Here's how the part is built. I have some questions about the finished solid (model axes, mm). Face numbers are marked on the shaded views. Coordinates: 2 decimals unless noted, no trailing zeros. Write each loop counter-clockwise with the first axis right and the second up, starting at its lowest first coordinate (ties: lowest second). Pieces come first, ordered by that corner, then holes. Notation, with made-up numbers: (73, 74) -> (80, 74) arc R20 cw to (80, 83) -> close; hole circle Ø6 at (23, 59). An arc over 180 degrees is marked (long way). Put each result on its own line as item: value. Start each with the question number.
Item 1: For pin 1 (3.5 mm diameter, centred on x = 9, z = -5.5, fed in from -Y), with a flat end and sliding along its axis, tell me the tip position at first contact or that it passes through.
Item 2: I want a section at C-C, the plane x = 0. List the corners of the cut face in (y, z) for me (3 decimals).
Item 3: I want a section at A-A, the plane z = 0. List the corners of the cut face in (x, y) for me (3 decimals), then the cut area to 3 significant figures.
Item 4: I want a section at D-D, the plane x = -9. State how many separate pieces and enclosed holes the cut face has, then the cut area to 3 significant figures.
Item 5: I need wall thicknesses on line 1 (Z direction, x = 16.5, y = 1.65); line 2 (X direction, y = 1.55, z = 0) (3 decimals); line 3 (X direction, y = 3.8, z = 9.25). Which ranges of each line are inside material? Lowest first, please. Write a range as [from, to].
Item 6: I want a section at B-B, the plane x = 14.5. List the corners of the cut face in (y, z) for me, then the cut area to 3 significant figures.
Item 7: If we mould it in two halves opening along X, with no side actions, what happens to the marked faces 1, 2 and 3? For each: released by +X, released by -X, zero draft, split by the parting line, or undercut.
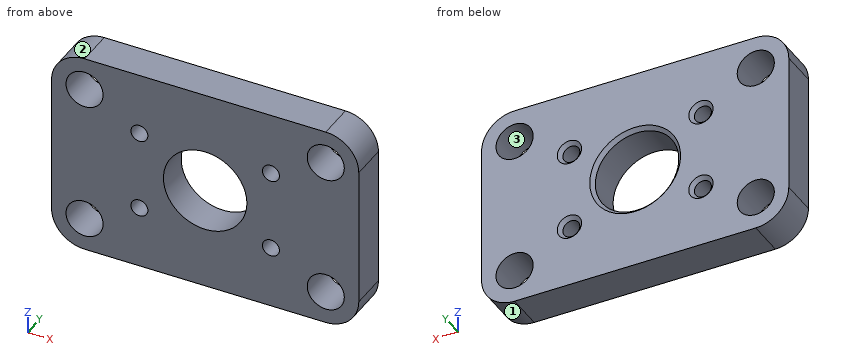
from build123d import *

# Parameters (mm, degrees)
SKETCH1_R           = 2.54
BOSS_EXTRUDE1_DEPTH = 5.08
SKETCH3_R           = 1.16205
SKETCH3_R_2         = 5.715
CUT_EXTRUDE4_DEPTH  = 6.08
CHAMFER1_SIZE       = 0.5


with BuildPart() as part:
    # Sketch1 → Boss-Extrude1 (new body)
    with BuildSketch(Plane(origin=(0, 0, 0), x_dir=(1, 0, 0), z_dir=(0, 1, 0))):
        with BuildLine():
            Line((-16.51, -14.0462), (16.51, -14.0462))
            ThreePointArc((16.51, -14.0462), (19.706971179, -12.721971179), (21.0312, -9.525))
            Line((21.0312, -9.525), (21.0312, 9.525))
            ThreePointArc((21.0312, 9.525), (19.706971179, 12.721971179), (16.51, 14.0462))
            Line((16.51, 14.0462), (-16.51, 14.0462))
            ThreePointArc((-16.51, 14.0462), (-19.706971179, 12.721971179), (-21.0312, 9.525))
            Line((-21.0312, 9.525), (-21.0312, -9.525))
            ThreePointArc((-21.0312, -9.525), (-19.706971179, -12.721971179), (-16.51, -14.0462))
        make_face()
        with Locations((-16.51, 9.525)):
            Circle(SKETCH1_R, mode=Mode.SUBTRACT)
        with Locations((-16.51, -9.525)):
            Circle(SKETCH1_R, mode=Mode.SUBTRACT)
        with Locations((16.51, -9.525)):
            Circle(SKETCH1_R, mode=Mode.SUBTRACT)
        with Locations((16.51, 9.525)):
            Circle(SKETCH1_R, mode=Mode.SUBTRACT)
    extrude(amount=BOSS_EXTRUDE1_DEPTH)

    # Sketch3 → Cut-Extrude4 (cut, through all)
    with BuildSketch(Plane(origin=(0, 5.08, 0), x_dir=(1, 0, 0), z_dir=(0, 1, 0))):
        with Locations((-9.0043, 5.4991)):
            Circle(SKETCH3_R)
        with Locations((9.0043, 5.4991)):
            Circle(SKETCH3_R)
        with Locations((9.0043, -5.4991)):
            Circle(SKETCH3_R)
        with Locations((-9.0043, -5.4991)):
            Circle(SKETCH3_R)
        Circle(SKETCH3_R_2)
    extrude(amount=-CUT_EXTRUDE4_DEPTH, mode=Mode.SUBTRACT)

    # Chamfer1
    chamfer1_edges = [part.edges().sort_by_distance(p)[0] for p in [
        (-5.715, 5.08, 0),
        (-10.16635, 5.08, 5.4991),
        (7.84225, 5.08, 5.4991),
        (7.84225, 5.08, -5.4991),
        (-10.16635, 5.08, -5.4991),
    ]]
    chamfer(chamfer1_edges, length=CHAMFER1_SIZE)


solid = part.part
Calculated:
1. pin 1: stops at y = 0
2. outline: (0, -14.046) -> (5.08, -14.046) -> (5.08, -6.215) -> (4.58, -5.715) -> (0, -5.715) -> close; (0, 5.715) -> (4.58, 5.715) -> (5.08, 6.215) -> (5.08, 14.046) -> (0, 14.046) -> close
3. outline: (-21.031, 0) -> (-5.715, 0) -> (-5.715, 4.58) -> (-6.215, 5.08) -> (-21.031, 5.08) -> close; (5.715, 0) -> (21.031, 0) -> (21.031, 5.08) -> (6.215, 5.08) -> (5.715, 4.58) -> close
3. area: 155 mm2
4. separate pieces: 3
4. enclosed holes: 0
4. area: 119 mm2
5. line 1: z = [-14.05, -12.06], [-6.99, 6.99], [12.06, 14.05]
5. line 2: x = [-21.031, -5.715], [5.715, 21.031]
5. line 3: x = [-21.03, -19.04], [-13.98, 13.98], [19.04, 21.03]
6. outline: (0, -14.05) -> (5.08, -14.05) -> (5.08, -11.08) -> (0, -11.08) -> close; (0, -7.97) -> (5.08, -7.97) -> (5.08, 7.97) -> (0, 7.97) -> close; (0, 11.08) -> (5.08, 11.08) -> (5.08, 14.05) -> (0, 14.05) -> close
6. area: 111 mm2
7. face 1: released by +X
7. face 2: released by -X
7. face 3: undercut
